```python
from build123d import *

# Parameters (mm, degrees)
BOSS_EXTRUDE1_DEPTH = 19
SKETCH2_R           = 1.63
CUT_EXTRUDE1_DEPTH  = 32.4
FILLET1_R           = 5
SKETCH4_R           = 3
CUT_EXTRUDE3_DEPTH  = 32.4


with BuildPart() as part:
    # Sketch1 → Boss-Extrude1 (new body, symmetric)
    with BuildSketch(Plane.XY):
        Polygon((-15.7, 80), (-12.7, 80), (-12.7, 4), (12.7, 4), (12.7, 80), (15.7, 80), (15.7, 0), (-15.7, 0), align=None)
    extrude(amount=BOSS_EXTRUDE1_DEPTH, both=True)

    # Sketch2 → Cut-Extrude1 (cut, through all)
    with BuildSketch(Plane(origin=(15.7, 0, 0), x_dir=(0, 0, -1), z_dir=(1, 0, 0))):
        with Locations((-7.75, 75.63)):
            Circle(SKETCH2_R)
        with Locations((7.75, 75.63)):
            Circle(SKETCH2_R)
        with Locations((-15.5, 62.2)):
            Circle(SKETCH2_R)
        with Locations((15.5, 62.2)):
            Circle(SKETCH2_R)
        with Locations((-7.75, 48.77)):
            Circle(SKETCH2_R)
        with Locations((7.75, 48.77)):
            Circle(SKETCH2_R)
    extrude(amount=-CUT_EXTRUDE1_DEPTH, mode=Mode.SUBTRACT)

    # Fillet1
    fillet1_edges = [part.edges().sort_by_distance(p)[0] for p in [
        (14.2, 80, -19),
        (15.7, 0, 0),
        (-15.7, 0, 0),
        (14.2, 80, 19),
        (-14.2, 80, 19),
        (-14.2, 80, -19),
    ]]
    fillet(fillet1_edges, radius=FILLET1_R)

    # Sketch4 → Cut-Extrude3 (cut, through all)
    with BuildSketch(Plane(origin=(15.7, 0, 0), x_dir=(0, 0, -1), z_dir=(1, 0, 0))):
        with Locations((0, 16.7)):
            Circle(SKETCH4_R)
    extrude(amount=-CUT_EXTRUDE3_DEPTH, mode=Mode.SUBTRACT)


solid = part.part
```
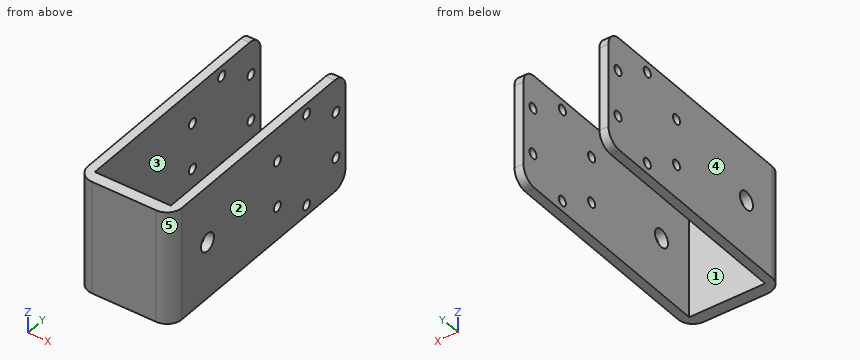
Input: part model. Units: mm. Frame: model coordinates. Face numbers are marked on the shaded views. A direction names the side the tool comes from. Give positions to 0.01 mm unless a question says otherwise; leave off trailing zeros. Loops run counter-clockwise (first coordinate to the right, second up) from the corner with the lowest first, then second, coordinate; pieces in that order, holes last. Notation, with made-up numbers: (-35.75, 17.5) -> (0.25, 17.5) arc R23 ccw to (0.25, 56.5) -> close; hole circle Ø2 at (-15, 17.25). An arc over 180 degrees is marked (long way). Use a Markdown table: item, result.
Q1. Section query A-A, the plane z = -7.75. Return the cut outline in (x, y).
Entries:
| item | result |
|---|---|
| outline | (-15.7, 5) arc R5 ccw to (-10.7, 0) -> (10.7, 0) arc R5 ccw to (15.7, 5) -> (15.7, 47.14) -> (12.7, 47.14) -> (12.7, 4) -> (-12.7, 4) -> (-12.7, 47.14) -> (-15.7, 47.14) -> close; (-15.7, 50.4) -> (-12.7, 50.4) -> (-12.7, 74) -> (-15.7, 74) -> close; (-15.7, 77.26) -> (-12.7, 77.26) -> (-12.7, 80) -> (-15.7, 80) -> close; (12.7, 50.4) -> (15.7, 50.4) -> (15.7, 74) -> (12.7, 74) -> close; (12.7, 77.26) -> (15.7, 77.26) -> (15.7, 80) -> (12.7, 80) -> close |
Q2. Section query C-C, the plane y = 48.77. Return the cut outline in (x, z), plus the area to 3 significant figures.
Entries:
| item | result |
|---|---|
| outline | (-15.7, -19) -> (-12.7, -19) -> (-12.7, -9.38) -> (-15.7, -9.38) -> close; (-15.7, -6.12) -> (-12.7, -6.12) -> (-12.7, 6.12) -> (-15.7, 6.12) -> close; (-15.7, 9.38) -> (-12.7, 9.38) -> (-12.7, 19) -> (-15.7, 19) -> close; (12.7, -19) -> (15.7, -19) -> (15.7, -9.38) -> (12.7, -9.38) -> close; (12.7, -6.12) -> (15.7, -6.12) -> (15.7, 6.12) -> (12.7, 6.12) -> close; (12.7, 9.38) -> (15.7, 9.38) -> (15.7, 19) -> (12.7, 19) -> close |
| area | 189 mm² |
Q3. Section query D-D, the plane z = 15.5. Return the cut outline in (x, y), plus the area to 3 significant figures.
Entries:
| item | result |
|---|---|
| outline | (-15.7, 5) arc R5 ccw to (-10.7, 0) -> (10.7, 0) arc R5 ccw to (15.7, 5) -> (15.7, 60.57) -> (12.7, 60.57) -> (12.7, 4) -> (-12.7, 4) -> (-12.7, 60.57) -> (-15.7, 60.57) -> close; (-15.7, 63.83) -> (-12.7, 63.83) -> (-12.7, 79.77) -> (-15.7, 79.77) -> close; (12.7, 63.83) -> (15.7, 63.83) -> (15.7, 79.77) -> (12.7, 79.77) -> close |
| area | 550 mm² |
Q4. Section query B-B, the plane y = 59. Return the cut outline in (x, z).
Entries:
| item | result |
|---|---|
| outline | (-15.7, -19) -> (-12.7, -19) -> (-12.7, 19) -> (-15.7, 19) -> close; (12.7, -19) -> (15.7, -19) -> (15.7, 19) -> (12.7, 19) -> close |
Q5. Pull-direction query (X, two-part tool) for the marked faces 3, 4 and 5; classes: pulls with the +X half, pulls with the -X half, needs draft (parallel to the pull), parting line crosses it, or undercut.
Entries:
| item | result |
|---|---|
| face 3 | undercut |
| face 4 | pulls with the -X half |
| face 5 | pulls with the +X half |
Q6. Ray query, probe 1 along Z at (x, y) = (13, 62); probe 2 along X at (y, z) = (19.5, -14.5); probe 3 along Y at (x, z) = (-13.5, -6.5). Return the intervals inside material, ascending. Write a range as from..to.
Entries:
| item | result |
|---|---|
| probe 1 | z = -19..-17.12, -13.88..13.88, 17.12..19 |
| probe 2 | x = -15.7..-12.7, 12.7..15.7 |
| probe 3 | y = 0.86..47.72, 49.82..74.58, 76.68..80 |
Q7. Access query for the marked faces 1 and 2. Directions: +Z, -Z, +X, -X, +Y, -Y. A direction counts if a zero-diameter tool reaches every point of the face in a straight line with its end or side. Return the directions, or none.
Entries:
| item | result |
|---|---|
| face 1 | +Z, -Z, +Y |
| face 2 | +Z, -Z, +X, +Y, -Y |
Q8. First-contact query: P1, Ø3, axis at y = 75.63, z = -7.75, coming from the +X side; P2, Ø10, axis at x = 7.5, z = -8.5, coming from the +Y side. Flat tips, straight axial feed; report the tip coordinate or a pass-through.
Entries:
| item | result |
|---|---|
| P1 | passes through |
| P2 | stops at y = 4 |
